Geometry check sheet. Reference: the model listing, model coordinates, mm. Face numbers are marked on the shaded views. A direction names the side the tool comes from. Round coordinates to 2 decimals unless told otherwise and drop trailing zeros. Write each loop counter-clockwise with the first axis right and the second up, starting at its lowest first coordinate (ties: lowest second). Pieces come first, ordered by that corner, then holes.
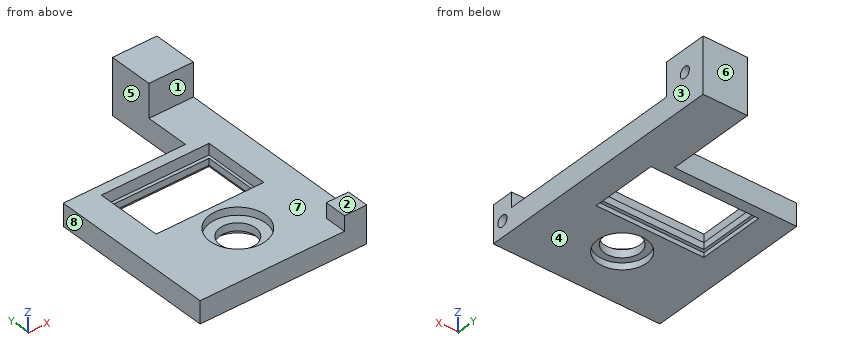
from build123d import *

# Parameters (mm, degrees)
SKETCH_1_W                      = 75
SKETCH_1_H                      = 115
EXTRUDE_1_DEPTH                 = 10
CUT_EXTRUDE_1_REACH             = 71.372
SKETCH_2_R                      = 8
SKETCH_3_R                      = 12.5
CUT_EXTRUDE_2_DEPTH             = 3.5
SKETCH_4_R                      = 11
CUT_EXTRUDE_3_DEPTH             = 3
SKETCH_6_W                      = 20
SKETCH_6_H                      = 20
EXTRUDE_2_DEPTH                 = 15
SKETCH_7_W                      = 6.681785618
SKETCH_7_H                      = 10
EXTRUDE_3_DEPTH                 = 10
CUT_EXTRUDE_4_REACH             = 75.058
SKETCH_8_W                      = 55
SKETCH_8_H                      = 40
CUT_EXTRUDE_4_DIRECTION_2_DEPTH = 74.058195981
CUT_EXTRUDE_5_REACH             = 75.058
SKETCH_9_W                      = 46
SKETCH_9_H                      = 27
SKETCH_10_W                     = 48.5
SKETCH_10_H                     = 30
CUT_EXTRUDE_6_DEPTH             = 2
SKETCH_11_W                     = 48.5
SKETCH_11_H                     = 30
CUT_EXTRUDE_7_DEPTH             = 5
SKETCH_12_R                     = 2.5
CUT_EXTRUDE_8_DEPTH             = 15


with BuildPart() as part:
    # 草图1 → 凸台-拉伸1 (new body)
    with BuildSketch(Plane.XY):
        Rectangle(SKETCH_1_W, SKETCH_1_H)
    extrude(amount=EXTRUDE_1_DEPTH)

    # 草图2 → 切除-拉伸1 (cut, up to next)
    with BuildSketch(Plane.XY.offset(10), mode=Mode.PRIVATE) as cut_extrude_1_sk1:
        with Locations((0, -32.5)):
            Circle(SKETCH_2_R)
    cut_extrude_1_tool1 = extrude(cut_extrude_1_sk1.sketch, amount=-CUT_EXTRUDE_1_REACH, mode=Mode.PRIVATE) & part.part
    add(cut_extrude_1_tool1.solids().sort_by_distance((0, -32.5, 10))[0], mode=Mode.SUBTRACT)

    # 草图3 → 切除-拉伸2 (cut)
    with BuildSketch(Plane.XY.offset(10)):
        with Locations((0, -32.5)):
            Circle(SKETCH_3_R)
    extrude(amount=-CUT_EXTRUDE_2_DEPTH, mode=Mode.SUBTRACT)

    # 草图4 → 切除-拉伸3 (cut)
    with BuildSketch(Plane(origin=(0, 0, 0), x_dir=(-1, 0, 0), z_dir=(0, 0, -1))):
        with Locations((0, -32.5)):
            Circle(SKETCH_4_R)
    extrude(amount=-CUT_EXTRUDE_3_DEPTH, mode=Mode.SUBTRACT)

    # 草图6 → 凸台-拉伸2 (add)
    with BuildSketch(Plane.XY.offset(10)):
        with Locations((27.5, 47.5)):
            Rectangle(SKETCH_6_W, SKETCH_6_H)
    extrude(amount=EXTRUDE_2_DEPTH)

    # 草图7 → 凸台-拉伸3 (add)
    with BuildSketch(Plane(origin=(37.5, 0, 0), x_dir=(0, 0, -1), z_dir=(1, 0, 0))):
        with Locations((-13.340892809, -52.5)):
            Rectangle(SKETCH_7_W, SKETCH_7_H)
    extrude(amount=-EXTRUDE_3_DEPTH)

    # 草图8 → 切除-拉伸4 (cut, up to next)
    with BuildSketch(Plane(origin=(0, 0, 0), x_dir=(-1, 0, 0), z_dir=(0, 0, -1)), mode=Mode.PRIVATE) as cut_extrude_4_sk1:
        with Locations((10, 37.5)):
            Rectangle(SKETCH_8_W, SKETCH_8_H)
    cut_extrude_4_tool1 = extrude(cut_extrude_4_sk1.sketch, amount=-CUT_EXTRUDE_4_REACH, mode=Mode.PRIVATE) & part.part
    add(cut_extrude_4_tool1.solids().sort_by_distance((-10, 37.5, 0))[0], mode=Mode.SUBTRACT)

    # 草图8 → 切除-拉伸4 direction 2 (cut)
    with BuildSketch(Plane(origin=(0, 0, 0), x_dir=(-1, 0, 0), z_dir=(0, 0, -1))):
        with Locations((10, 37.5)):
            Rectangle(SKETCH_8_W, SKETCH_8_H)
    extrude(amount=CUT_EXTRUDE_4_DIRECTION_2_DEPTH, mode=Mode.SUBTRACT)

    # 草图9 → 切除-拉伸5 (cut, up to next)
    with BuildSketch(Plane(origin=(0, 0, 0), x_dir=(-1, 0, 0), z_dir=(0, 0, -1)), mode=Mode.PRIVATE) as cut_extrude_5_sk1:
        with Locations((0, -2.234079676)):
            Rectangle(SKETCH_9_W, SKETCH_9_H)
    cut_extrude_5_tool1 = extrude(cut_extrude_5_sk1.sketch, amount=-CUT_EXTRUDE_5_REACH, mode=Mode.PRIVATE) & part.part
    add(cut_extrude_5_tool1.solids().sort_by_distance((0, -2.23408, 0))[0], mode=Mode.SUBTRACT)

    # 草图10 → 切除-拉伸6 (cut)
    with BuildSketch(Plane(origin=(0, 0, 0), x_dir=(-1, 0, 0), z_dir=(0, 0, -1))):
        with Locations((0, -2.234079676)):
            Rectangle(SKETCH_10_W, SKETCH_10_H)
    extrude(amount=-CUT_EXTRUDE_6_DEPTH, mode=Mode.SUBTRACT)

    # 草图11 → 切除-拉伸7 (cut)
    with BuildSketch(Plane.XY.offset(10)):
        with Locations((0, -2.234079676)):
            Rectangle(SKETCH_11_W, SKETCH_11_H)
    extrude(amount=-CUT_EXTRUDE_7_DEPTH, mode=Mode.SUBTRACT)

    # 草图12 → 切除-拉伸8 (cut)
    with BuildSketch(Plane(origin=(37.5, 0, 0), x_dir=(0, 0, -1), z_dir=(1, 0, 0))):
        with Locations((-15, 47.5)):
            Circle(SKETCH_12_R)
        with Locations((-7, -52.5)):
            Circle(SKETCH_12_R)
    extrude(amount=-CUT_EXTRUDE_8_DEPTH, mode=Mode.SUBTRACT)


solid = part.part
1. Release check for a two-part mould opening along Y. For the marked faces 6, 7 and 8 record: +Y half, -Y half, draft (parallel to the pull), parting line (faces both ways), or undercut.
2. Section check B-B (x = -16.5). Record the cut outline in (y, z), plus the area to 3 significant figures.
3. Scan lines: line 1 along Y through (x, z) = (31, 15); line 2 along Y through (x, z) = (0, 8.7); line 3 along X through (y, z) = (-8, 9.5). Record each from-to range of solid material in increasing order.
4. Section check C-C (z = 15). Record the cut outline in (x, y), plus the area to 3 significant figures.
5. Access from +Z, -Z, +X, -X, +Y, -Y to the whole of each face (thin tool, end or side, straight path). Record for the marked faces 1, 2, 3, 4 and 5.
6. Section check D-D (x = 29.5). Record the cut outline in (y, z).
7. Depth check by flat-ended pin: pin 1 Ø1.5 at (x, y) = (21, 14.5) entering from +Z; pin 2 Ø4.5 at (y, z) = (47.5, 15) entering from +X; pin 3 Ø3.5 at (x, z) = (-8.5, 3) entering from +Y; pin 4 Ø6 at (y, z) = (6, 14) entering from +X. Enter the tip coordinate at first touch or a pass-through.
8. Section check A-A (y = 9.5). Record the cut outline in (x, z), plus the area to 4 significant figures.
Results below:
1. face 6: +Y half
1. face 7: undercut
1. face 8: draft
2. outline: (-57.5, 0) - (-17.23, 0) - (-17.23, 2) - (-15.73, 2) - (-15.73, 5) - (-17.23, 5) - (-17.23, 10) - (-57.5, 10) - close; (11.27, 2) - (12.77, 2) - (12.77, 0) - (17.5, 0) - (17.5, 10) - (12.77, 10) - (12.77, 5) - (11.27, 5) - close
2. area: 459 mm2
3. line 1: y = -57.5 to -47.5, 37.5 to 45, 50 to 57.5
3. line 2: y = -57.5 to -45, -20 to -17.23, 12.77 to 17.5
3. line 3: x = -37.5 to -24.25, 24.25 to 37.5
4. outline: (17.5, 37.5) - (37.5, 37.5) - (37.5, 45) - (22.5, 45) - (22.5, 50) - (37.5, 50) - (37.5, 57.5) - (17.5, 57.5) - close; (27.5, -57.5) - (37.5, -57.5) - (37.5, -47.5) - (27.5, -47.5) - close
4. area: 425 mm2
5. face 1: +Z, +X, -X
5. face 2: +Z, +X, -X, -Y
5. face 3: +Z, -Z, +X, +Y, -Y
5. face 4: -Z, +X, -X, +Y, -Y
5. face 5: +Z, -Z, -X, +Y
6. outline: (-57.5, 0) - (57.5, 0) - (57.5, 25) - (37.5, 25) - (37.5, 10) - (-47.5, 10) - (-47.5, 16.68) - (-57.5, 16.68) - close; hole circle Ø5 at (-52.5, 7); hole circle Ø5 at (47.5, 15)
7. pin 1: stops at z = 10
7. pin 2: stops at x = 22.5
7. pin 3: stops at y = 17.5
7. pin 4: passes through
8. outline: (-37.5, 0) - (-24.25, 0) - (-24.25, 2) - (-23, 2) - (-23, 5) - (-24.25, 5) - (-24.25, 10) - (-37.5, 10) - close; (23, 2) - (24.25, 2) - (24.25, 0) - (37.5, 0) - (37.5, 10) - (24.25, 10) - (24.25, 5) - (23, 5) - close
8. area: 272.5 mm2
